```python
from build123d import *

# Parameters (mm, degrees)
SKETCH1_R           = 3.55
SKETCH1_R_2         = 1.25
BOSS_EXTRUDE1_DEPTH = 2.3
BOSS_EXTRUDE2_START = 2.3
SKETCH1_3_R         = 3.55
SKETCH1_3_R_2       = 1.25
BOSS_EXTRUDE2_DEPTH = 1.85
BOSS_EXTRUDE3_START = 2.3
BOSS_EXTRUDE3_DEPTH = 9
CUT_EXTRUDE3_REACH  = 73.238
SKETCH2_W           = 7.938
SKETCH2_H           = 8.3
CUT_EXTRUDE4_REACH  = 73.092
SKETCH3_W           = 13.048
SKETCH3_H           = 6.12
CUT_EXTRUDE5_REACH  = 73.092
SKETCH4_W           = 12.28
SKETCH4_H           = 7.81


with BuildPart() as part:
    # Sketch1 → Boss-Extrude1 (new body)
    # profile 1 of 7: a face of its own
    with BuildSketch(Plane(origin=(0, 0, 0), x_dir=(1, 0, 0), z_dir=(0, 1, 0))):
        with BuildLine():
            ThreePointArc((-3.5, -3.556), (-1.433345448, 1.433345448), (3.556, 3.5))
            Line((3.556, 3.5), (42.304, 3.5))
            ThreePointArc((42.304, 3.5), (47.293345448, 1.433345448), (49.36, -3.556))
            Line((49.36, -3.556), (49.36, -39.344))
            ThreePointArc((49.36, -39.344), (47.293345448, -44.333345448), (42.304, -46.4))
            Line((42.304, -46.4), (3.556, -46.4))
            ThreePointArc((3.556, -46.4), (-1.433345448, -44.333345448), (-3.5, -39.344))
            Line((-3.5, -39.344), (-3.5, -3.556))
        make_face()
        with BuildLine():
            Line((-0.5, -3.556), (-0.5, -39.344))
            ThreePointArc((-0.5, -39.344), (0.687974896, -42.212025104), (3.556, -43.4))
            Line((3.556, -43.4), (42.304, -43.4))
            ThreePointArc((42.304, -43.4), (45.172025104, -42.212025104), (46.36, -39.344))
            Line((46.36, -39.344), (46.36, -3.556))
            ThreePointArc((46.36, -3.556), (45.172025104, -0.687974896), (42.304, 0.5))
            Line((42.304, 0.5), (3.556, 0.5))
            ThreePointArc((3.556, 0.5), (0.687974896, -0.687974896), (-0.5, -3.556))
        make_face(mode=Mode.SUBTRACT)
    # profile 2 of 7: a face of its own
    with BuildSketch(Plane(origin=(0, 0, 0), x_dir=(1, 0, 0), z_dir=(0, 1, 0))):
        with BuildLine():
            ThreePointArc((-0.5, -3.556), (0.687974896, -0.687974896), (3.556, 0.5))
            Line((3.556, 0.5), (42.304, 0.5))
            ThreePointArc((42.304, 0.5), (45.172025104, -0.687974896), (46.36, -3.556))
            Line((46.36, -3.556), (46.36, -39.344))
            ThreePointArc((46.36, -39.344), (45.172025104, -42.212025104), (42.304, -43.4))
            Line((42.304, -43.4), (3.556, -43.4))
            ThreePointArc((3.556, -43.4), (0.687974896, -42.212025104), (-0.5, -39.344))
            Line((-0.5, -39.344), (-0.5, -3.556))
        make_face()
        with BuildLine():
            Line((0, -3.556), (0, -39.344))
            ThreePointArc((0, -39.344), (1.041528286, -41.858471714), (3.556, -42.9))
            Line((3.556, -42.9), (42.304, -42.9))
            ThreePointArc((42.304, -42.9), (44.818471714, -41.858471714), (45.86, -39.344))
            Line((45.86, -39.344), (45.86, -3.556))
            ThreePointArc((45.86, -3.556), (44.818471714, -1.041528286), (42.304, 0))
            Line((42.304, 0), (3.556, 0))
            ThreePointArc((3.556, 0), (1.041528286, -1.041528286), (0, -3.556))
        make_face(mode=Mode.SUBTRACT)
    # profile 3 of 7: a face of its own
    with BuildSketch(Plane(origin=(0, 0, 0), x_dir=(1, 0, 0), z_dir=(0, 1, 0))):
        with BuildLine():
            ThreePointArc((0, -3.556), (1.041528286, -1.041528286), (3.556, 0))
            Line((3.556, 0), (42.304, 0))
            ThreePointArc((42.304, 0), (44.818471714, -1.041528286), (45.86, -3.556))
            Line((45.86, -3.556), (45.86, -39.344))
            ThreePointArc((45.86, -39.344), (44.818471714, -41.858471714), (42.304, -42.9))
            Line((42.304, -42.9), (3.556, -42.9))
            ThreePointArc((3.556, -42.9), (1.041528286, -41.858471714), (0, -39.344))
            Line((0, -39.344), (0, -3.556))
        make_face()
        with Locations((3.556, -39.344)):
            Circle(SKETCH1_R, mode=Mode.SUBTRACT)
        with Locations((42.304, -39.344)):
            Circle(SKETCH1_R, mode=Mode.SUBTRACT)
        with Locations((42.304, -3.556)):
            Circle(SKETCH1_R, mode=Mode.SUBTRACT)
        with Locations((3.556, -3.556)):
            Circle(SKETCH1_R, mode=Mode.SUBTRACT)
    # profile 4 of 7: a face of its own
    with BuildSketch(Plane(origin=(0, 0, 0), x_dir=(1, 0, 0), z_dir=(0, 1, 0))):
        with Locations((42.304, -39.344)):
            Circle(SKETCH1_R)
        with Locations(Location((42.304, -39.344, 0), (0, 0, 270))):
            Circle(SKETCH1_R_2, mode=Mode.SUBTRACT)
    # profile 5 of 7: a face of its own
    with BuildSketch(Plane(origin=(0, 0, 0), x_dir=(1, 0, 0), z_dir=(0, 1, 0))):
        with Locations((3.556, -39.344)):
            Circle(SKETCH1_R)
        with Locations(Location((3.556, -39.344, 0), (0, 0, 270))):
            Circle(SKETCH1_R_2, mode=Mode.SUBTRACT)
    # profile 6 of 7: a face of its own
    with BuildSketch(Plane(origin=(0, 0, 0), x_dir=(1, 0, 0), z_dir=(0, 1, 0))):
        with Locations((3.556, -3.556)):
            Circle(SKETCH1_R)
        with Locations(Location((3.556, -3.556, 0), (0, 0, 270))):
            Circle(SKETCH1_R_2, mode=Mode.SUBTRACT)
    # profile 7 of 7: a face of its own
    with BuildSketch(Plane(origin=(0, 0, 0), x_dir=(1, 0, 0), z_dir=(0, 1, 0))):
        with Locations((42.304, -3.556)):
            Circle(SKETCH1_R)
        with Locations(Location((42.304, -3.556, 0), (0, 0, 270))):
            Circle(SKETCH1_R_2, mode=Mode.SUBTRACT)
    extrude(amount=BOSS_EXTRUDE1_DEPTH)

    # Sketch1<3> → Boss-Extrude2 (add)
    # profile 1 of 4: a face of its own
    with BuildSketch(Plane(origin=(0, 0, 0), x_dir=(1, 0, 0), z_dir=(0, 1, 0)).offset(BOSS_EXTRUDE2_START)):
        with Locations(Location((3.556, -3.556, 0), (0, 0, 270))):
            Circle(SKETCH1_3_R)
        with Locations(Location((3.556, -3.556, 0), (0, 0, 270))):
            Circle(SKETCH1_3_R_2, mode=Mode.SUBTRACT)
    # profile 2 of 4: a face of its own
    with BuildSketch(Plane(origin=(0, 0, 0), x_dir=(1, 0, 0), z_dir=(0, 1, 0)).offset(BOSS_EXTRUDE2_START)):
        with Locations(Location((42.304, -3.556, 0), (0, 0, 270))):
            Circle(SKETCH1_3_R)
        with Locations(Location((42.304, -3.556, 0), (0, 0, 270))):
            Circle(SKETCH1_3_R_2, mode=Mode.SUBTRACT)
    # profile 3 of 4: a face of its own
    with BuildSketch(Plane(origin=(0, 0, 0), x_dir=(1, 0, 0), z_dir=(0, 1, 0)).offset(BOSS_EXTRUDE2_START)):
        with Locations(Location((42.304, -39.344, 0), (0, 0, 270))):
            Circle(SKETCH1_3_R)
        with Locations(Location((42.304, -39.344, 0), (0, 0, 270))):
            Circle(SKETCH1_3_R_2, mode=Mode.SUBTRACT)
    # profile 4 of 4: a face of its own
    with BuildSketch(Plane(origin=(0, 0, 0), x_dir=(1, 0, 0), z_dir=(0, 1, 0)).offset(BOSS_EXTRUDE2_START)):
        with Locations(Location((3.556, -39.344, 0), (0, 0, 270))):
            Circle(SKETCH1_3_R)
        with Locations(Location((3.556, -39.344, 0), (0, 0, 270))):
            Circle(SKETCH1_3_R_2, mode=Mode.SUBTRACT)
    extrude(amount=BOSS_EXTRUDE2_DEPTH)

    # Sketch1<4> → Boss-Extrude3 (add)
    with BuildSketch(Plane(origin=(0, 0, 0), x_dir=(1, 0, 0), z_dir=(0, 1, 0)).offset(BOSS_EXTRUDE3_START)):
        with BuildLine():
            ThreePointArc((-3.5, -3.556), (-1.433345448, 1.433345448), (3.556, 3.5))
            Line((3.556, 3.5), (42.304, 3.5))
            ThreePointArc((42.304, 3.5), (47.293345448, 1.433345448), (49.36, -3.556))
            Line((49.36, -3.556), (49.36, -39.344))
            ThreePointArc((49.36, -39.344), (47.293345448, -44.333345448), (42.304, -46.4))
            Line((42.304, -46.4), (3.556, -46.4))
            ThreePointArc((3.556, -46.4), (-1.433345448, -44.333345448), (-3.5, -39.344))
            Line((-3.5, -39.344), (-3.5, -3.556))
        make_face()
        with BuildLine():
            Line((-0.5, -3.556), (-0.5, -39.344))
            ThreePointArc((-0.5, -39.344), (0.687974896, -42.212025104), (3.556, -43.4))
            Line((3.556, -43.4), (42.304, -43.4))
            ThreePointArc((42.304, -43.4), (45.172025104, -42.212025104), (46.36, -39.344))
            Line((46.36, -39.344), (46.36, -3.556))
            ThreePointArc((46.36, -3.556), (45.172025104, -0.687974896), (42.304, 0.5))
            Line((42.304, 0.5), (3.556, 0.5))
            ThreePointArc((3.556, 0.5), (0.687974896, -0.687974896), (-0.5, -3.556))
        make_face(mode=Mode.SUBTRACT)
    extrude(amount=BOSS_EXTRUDE3_DEPTH)

    # Sketch2 → Cut-Extrude3 (cut, up to next)
    with BuildSketch(Plane(origin=(49.36, 0, 0), x_dir=(0, 0, -1), z_dir=(1, 0, 0)), mode=Mode.PRIVATE) as cut_extrude3_sk1:
        with Locations((-26.725, 7.15)):
            Rectangle(SKETCH2_W, SKETCH2_H)
    cut_extrude3_tool1 = extrude(cut_extrude3_sk1.sketch, amount=-CUT_EXTRUDE3_REACH, mode=Mode.PRIVATE) & part.part
    add(cut_extrude3_tool1.solids().sort_by_distance((49.36, 7.15, 26.725))[0], mode=Mode.SUBTRACT)

    # Sketch3 → Cut-Extrude4 (cut, up to next)
    with BuildSketch(Plane.XY.offset(46.4), mode=Mode.PRIVATE) as cut_extrude4_sk1:
        with Locations((13.58, 8.24)):
            Rectangle(SKETCH3_W, SKETCH3_H)
    cut_extrude4_tool1 = extrude(cut_extrude4_sk1.sketch, amount=-CUT_EXTRUDE4_REACH, mode=Mode.PRIVATE) & part.part
    add(cut_extrude4_tool1.solids().sort_by_distance((13.58, 8.24, 46.4))[0], mode=Mode.SUBTRACT)

    # Sketch4 → Cut-Extrude5 (cut, up to next)
    with BuildSketch(Plane.XY.offset(46.4), mode=Mode.PRIVATE) as cut_extrude5_sk1:
        with Locations((25.394, 7.395)):
            Rectangle(SKETCH4_W, SKETCH4_H)
    cut_extrude5_tool1 = extrude(cut_extrude5_sk1.sketch, amount=-CUT_EXTRUDE5_REACH, mode=Mode.PRIVATE) & part.part
    add(cut_extrude5_tool1.solids().sort_by_distance((25.394, 7.395, 46.4))[0], mode=Mode.SUBTRACT)


solid = part.part
```
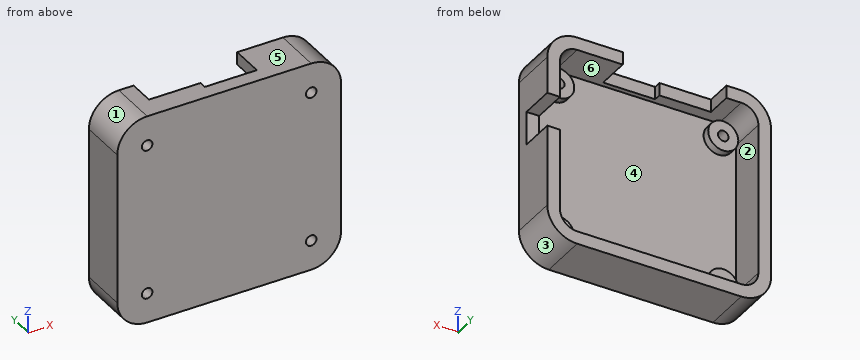
Design review of the part built by this model. Coordinates are the model's own, in mm. Face numbers are marked on the shaded views. A direction names the side the tool comes from. Coordinates: 2 decimals unless noted, no trailing zeros. Order: outer loops, then holes, each group sorted by start corner. A loop starts at its lowest first (then second) coordinate and runs counter-clockwise, first axis right, second up.
1) For the marked faces 5 and 6, list the 3-axis set-ups (+Z, -Z, +X, -X, +Y, -Y) from which the entire face can be reached by the end or side of a thin tool; tool diameter is ignored.
2) Take a section at A-A, the plane y = 9.75. Give the boundary of the cut face in (x, z).
3) Take a section at C-C, the plane z = 25. Give the boundary of the cut face in (x, y).
4) Mouldability with a two-part tool opening along Z and no side actions: class the marked faces 1, 2, 3 and 4 as +Z half, -Z half, draft (parallel to the pull), parting line (faces both ways), or undercut.
5) Clearance check with flat-ended pins moving along their axes: pin 1 (2 mm diameter, centred on x = 3, z = 39.5, fed in from +Y); pin 2 (1.5 mm diameter, centred on y = 8, z = 44.5, fed in from +X); pin 3 (1 mm diameter, centred on x = 19.5, z = 14, fed in from +Y). State where each tip first meets the part, or that it passes through.
6) Take a section at D-D, the plane x = 45. Give the boundary of the cut face in (y, z).
7) Wall thickness on line 1 along X through (y, z) = (9.5, 22); line 2 along Z through (x, y) = (44, 4); line 3 along Z through (x, y) = (3.5, 4.25): over which ranges is each line inside the solid? List them lowest first.
8) Take a section at B-B, the plane x = 8. Give the boundary of the cut face in (y, z).
Returned:
1. face 5: +Z, +X, -X, +Y, -Y
1. face 6: +Y
2. outline: (-3.5, 3.56) arc R7.06 ccw to (3.56, -3.5) - (42.3, -3.5) arc R7.06 ccw to (49.36, 3.56) - (49.36, 22.76) - (46.36, 22.76) - (46.36, 3.56) arc R4.06 cw to (42.3, -0.5) - (3.56, -0.5) arc R4.06 cw to (-0.5, 3.56) - (-0.5, 39.34) arc R4.06 cw to (3.56, 43.4) - (7.06, 43.4) - (7.06, 46.4) - (3.56, 46.4) arc R7.06 ccw to (-3.5, 39.34) - close; (31.53, 43.4) - (42.3, 43.4) arc R4.06 cw to (46.36, 39.34) - (46.36, 30.69) - (49.36, 30.69) - (49.36, 39.34) arc R7.06 ccw to (42.3, 46.4) - (31.53, 46.4) - close
3. outline: (-3.5, 0) - (49.36, 0) - (49.36, 3) - (46.36, 3) - (46.36, 2.3) - (-0.5, 2.3) - (-0.5, 11.3) - (-3.5, 11.3) - close
4. face 1: +Z half
4. face 2: undercut
4. face 3: -Z half
4. face 4: undercut
5. pin 1: stops at y = 4.15
5. pin 2: stops at x = 47.82
5. pin 3: stops at y = 2.3
6. outline: (0, -2.96) - (11.3, -2.96) - (11.3, 0.53) - (2.3, 0.53) - (2.3, 1.25) - (4.15, 1.25) - (4.15, 5.87) - (2.3, 5.87) - (2.3, 37.03) - (4.15, 37.03) - (4.15, 41.65) - (2.3, 41.65) - (2.3, 42.37) - (11.3, 42.37) - (11.3, 45.86) - (0, 45.86) - close
7. line 1: x = -3.5 to -0.5, 46.36 to 49.36
7. line 2: z = -3.29 to -0.13, 0.44 to 6.67, 36.23 to 42.46, 43.03 to 46.19
7. line 3: z = -3.5 to -0.5, 43.4 to 46.4
8. outline: (0, -3.5) - (11.3, -3.5) - (11.3, -0.5) - (2.3, -0.5) - (2.3, 43.4) - (5.18, 43.4) - (5.18, 46.4) - (0, 46.4) - close
